from build123d import *
from OCP.BRepFilletAPI import BRepFilletAPI_MakeChamfer

# Parameters (mm, degrees)
SZKIC1_W                    = 47
SZKIC1_H                    = 33
SZKIC1_R                    = 7.6
DODANIE_WYCI_GNI_CIE1_DEPTH = 5
SZKIC2_W                    = 7
SZKIC2_H                    = 20.6
DODANIE_WYCI_GNI_CIE2_DEPTH = 10
SFAZOWANIE1_SIZE            = 5
SFAZOWANIE1_SIZE2           = 2.886751346
SZKIC3_R                    = 2
WYTNIJ_WYCI_GNI_CIE1_DEPTH  = 46.131917752
ZAOKR_GLENIE1_R             = 1
SZKIC4_W                    = 11.5
SZKIC4_H                    = 3
SZKIC4_W_2                  = 12
SZKIC4_H_2                  = 2.980259267
DODANIE_WYCI_GNI_CIE3_DEPTH = 27.5
DODANIE_WYCI_GNI_CIE4_START = 3
SZKIC5_W                    = 20.6
SZKIC5_H                    = 20.6
DODANIE_WYCI_GNI_CIE4_DEPTH = 3


with BuildPart() as part:
    # Szkic1 → Dodanie-wyciągnięcie1 (new body)
    # profile 1 of 3: a face of its own
    with BuildSketch(Plane.XY):
        Rectangle(SZKIC1_W, SZKIC1_H)
        Circle(SZKIC1_R, mode=Mode.SUBTRACT)
    # profile 2 of 3: a face of its own
    with BuildSketch(Plane.XY):
        with BuildLine():
            Line((4.175823272, -6.35), (-4.175823272, -6.35))
            ThreePointArc((-4.175823272, -6.35), (0, -7.6), (4.175823272, -6.35))
        make_face()
    # profile 3 of 3: a face of its own
    with BuildSketch(Plane.XY):
        with BuildLine():
            ThreePointArc((4.175823272, 6.35), (0, 7.6), (-4.175823272, 6.35))
            Line((-4.175823272, 6.35), (4.175823272, 6.35))
        make_face()
    extrude(amount=DODANIE_WYCI_GNI_CIE1_DEPTH)

    # Szkic2 → Dodanie-wyciągnięcie2 (add)
    with BuildSketch(Plane(origin=(0, 0, 0), x_dir=(-1, 0, 0), z_dir=(0, 0, -1))):
        with Locations((-13.8, 0)):
            Rectangle(SZKIC2_W, SZKIC2_H)
        with Locations((13.8, 0)):
            Rectangle(SZKIC2_W, SZKIC2_H)
    extrude(amount=DODANIE_WYCI_GNI_CIE2_DEPTH)

    # Sfazowanie1: one chamfer whose edges measure the first distance from different faces: ONE call of the kernel's chamfer builder (chamfer() names one face for all edges)
    sfazowanie1_edges_1 = [part.edges().sort_by_distance(p)[0] for p in [
        (13.8, 10.3, -10),
    ]]
    sfazowanie1_side_1 = [part.faces().sort_by_distance(p)[0] for p in [
        (13.8, 10.3, -5),
    ]]
    sfazowanie1_edges_2 = [part.edges().sort_by_distance(p)[0] for p in [
        (13.8, -10.3, -10),
    ]]
    sfazowanie1_side_2 = [part.faces().sort_by_distance(p)[0] for p in [
        (13.8, -10.3, -5),
    ]]
    sfazowanie1_edges_3 = [part.edges().sort_by_distance(p)[0] for p in [
        (-13.8, 10.3, -10),
    ]]
    sfazowanie1_side_3 = [part.faces().sort_by_distance(p)[0] for p in [
        (-13.8, 10.3, -5),
    ]]
    sfazowanie1_edges_4 = [part.edges().sort_by_distance(p)[0] for p in [
        (-13.8, -10.3, -10),
    ]]
    sfazowanie1_side_4 = [part.faces().sort_by_distance(p)[0] for p in [
        (-13.8, -10.3, -5),
    ]]
    sfazowanie1 = BRepFilletAPI_MakeChamfer(part.part.solid().wrapped)
    for e in sfazowanie1_edges_1:
        sfazowanie1.Add(SFAZOWANIE1_SIZE, SFAZOWANIE1_SIZE2, e.wrapped, sfazowanie1_side_1[0].wrapped)  # the first distance lies on this face
    for e in sfazowanie1_edges_2:
        sfazowanie1.Add(SFAZOWANIE1_SIZE, SFAZOWANIE1_SIZE2, e.wrapped, sfazowanie1_side_2[0].wrapped)  # the first distance lies on this face
    for e in sfazowanie1_edges_3:
        sfazowanie1.Add(SFAZOWANIE1_SIZE, SFAZOWANIE1_SIZE2, e.wrapped, sfazowanie1_side_3[0].wrapped)  # the first distance lies on this face
    for e in sfazowanie1_edges_4:
        sfazowanie1.Add(SFAZOWANIE1_SIZE, SFAZOWANIE1_SIZE2, e.wrapped, sfazowanie1_side_4[0].wrapped)  # the first distance lies on this face
    add(Compound.cast(sfazowanie1.Shape()), mode=Mode.REPLACE)

    # Szkic3 → Wytnij-wyciągnięcie1 (cut, through all)
    with BuildSketch(Plane(origin=(17.3, 0, 0), x_dir=(0, 0, -1), z_dir=(1, 0, 0))):
        with Locations((5, 4.3)):
            Circle(SZKIC3_R)
        with Locations((5, -4.3)):
            Circle(SZKIC3_R)
    extrude(amount=-WYTNIJ_WYCI_GNI_CIE1_DEPTH, mode=Mode.SUBTRACT)

    # Zaokrąglenie1
    zaokr_glenie1_edges = [part.edges().sort_by_distance(p)[0] for p in [
        (-23.5, -16.5, 2.5),
        (-23.5, 16.5, 2.5),
        (23.5, 16.5, 2.5),
        (23.5, -16.5, 2.5),
    ]]
    fillet(zaokr_glenie1_edges, radius=ZAOKR_GLENIE1_R)

    # Szkic4 → Dodanie-wyciągnięcie3 (add)
    with BuildSketch(Plane(origin=(0, 0, 0), x_dir=(-1, 0, 0), z_dir=(0, 0, -1))):
        with Locations((-1.5, 15)):
            Rectangle(SZKIC4_W, SZKIC4_H)
        with Locations((-1.25, -15.009870366)):
            Rectangle(SZKIC4_W_2, SZKIC4_H_2)
    extrude(amount=DODANIE_WYCI_GNI_CIE3_DEPTH)

    # Szkic5 → Dodanie-wyciągnięcie4 (add)
    with BuildSketch(Plane(origin=(0, 0, 0), x_dir=(-1, 0, 0), z_dir=(0, 0, -1)).offset(DODANIE_WYCI_GNI_CIE4_START)):
        Rectangle(SZKIC5_W, SZKIC5_H)
        with BuildLine():
            Line((4.175823272, -6.35), (-4.175823272, -6.35))
            ThreePointArc((-4.175823272, -6.35), (-7.6, 0), (-4.175823272, 6.35))
            Line((-4.175823272, 6.35), (4.175823272, 6.35))
            ThreePointArc((4.175823272, 6.35), (7.6, 0), (4.175823272, -6.35))
        make_face(mode=Mode.SUBTRACT)
    extrude(amount=-DODANIE_WYCI_GNI_CIE4_DEPTH)


solid = part.part
Geometry check sheet. Reference: the model listing, model coordinates, mm. A direction names the side the tool comes from. Round coordinates to 2 decimals unless told otherwise and drop trailing zeros. Order: outer loops, then holes, each group sorted by start corner. A loop starts at its lowest first (then second) coordinate and runs counter-clockwise, first axis right, second up. Notation, with made-up numbers: M 12.25,84.25 L 20.25,84.25 A9 ccw 20.25,100.25 Z; hole C 84,54.25 d9. An arc over 180 degrees is marked long. Answer in a Markdown table with one row per item. Add a question column.
Item 1: Sectioned sample at A-A, the plane z = -24.5. Enter the section's corners in (x, y), plus the area to 3 significant figures.
Item 2: Material ranges on L1, parallel to Y at x = 1, z = -11.5; L2, parallel to Z at x = 18.5, y = -12; L3, parallel to Z at x = 12, y = -7, recorded low to high. Write a range as [from, to].
Item 3: Sectioned sample at D-D, the plane z = 2.5. Enter the section's corners in (x, y), plus the area to 3 significant figures.
Item 4: Depth check by flat-ended pin: pin 1 Ø1 at (x, y) = (0.5, 9.5) entering from -Z; pin 2 Ø7.5 at (y, z) = (3, -7.5) entering from +X; pin 3 Ø2 at (x, y) = (15, 0.5) entering from -Z; pin 4 Ø2 at (y, z) = (5, -5) entering from -X. Enter the tip coordinate at first touch or a pass-through.
Item 5: Draft check along Y on faces 1 (the face through (-23.215, -16.199, 2.535)), 2 (the face through (0, -10.3, -2)), 3 (the face through (-23.5, 0, 2)). Enter one of: released by +Y, released by -Y, zero draft, split by the parting line, or undercut.
Item 6: Sectioned sample at B-B, the plane z = -1.5. Enter the section's corners in (x, y), plus the area to 3 significant figures.
Item 7: Sectioned sample at C-C, the plane x = 1.5. Enter the section's corners in (y, z).
Item 8: Set-up check for faces 4 (the face through (23.199, 16.215, 2.535)), 5 (the face through (0, 10.3, -2)), 6 (the face through (-4.25, 15, -14)): record each of +Z, -Z, +X, -X, +Y, -Y from which the full face is reachable in a straight line by a thin tool's end or side.
Filled in:
| question | item | result |
|---|---|---|
| 1 | outline | M -4.75,-16.5 L 7.25,-16.5 L 7.25,-13.52 L -4.75,-13.52 Z; M -4.25,13.5 L 7.25,13.5 L 7.25,16.5 L -4.25,16.5 Z |
| 1 | area | 70.3 mm² |
| 2 | L1 | y = [-16.5, -13.52], [13.5, 16.5] |
| 2 | L2 | z = [0, 5] |
| 2 | L3 | z = [-10, 5] |
| 3 | outline | M -23.5,-15.5 A1 ccw -22.5,-16.5 L 22.5,-16.5 A1 ccw 23.5,-15.5 L 23.5,15.5 A1 ccw 22.5,16.5 L -22.5,16.5 A1 ccw -23.5,15.5 Z; hole M -4.18,-6.35 L 4.18,-6.35 A7.6 ccw 4.18,6.35 L -4.18,6.35 A7.6 ccw Z |
| 3 | area | 1,380 mm² |
| 4 | pin 1 | stops at z = -3 |
| 4 | pin 2 | stops at x = 17.3 |
| 4 | pin 3 | stops at z = -10 |
| 4 | pin 4 | passes through |
| 5 | face 1 | released by -Y |
| 5 | face 2 | undercut |
| 5 | face 3 | zero draft |
| 6 | outline | M -17.3,-10.3 L 17.3,-10.3 L 17.3,10.3 L -17.3,10.3 Z; M -4.75,-16.5 L 7.25,-16.5 L 7.25,-13.52 L -4.75,-13.52 Z; M -4.25,13.5 L 7.25,13.5 L 7.25,16.5 L -4.25,16.5 Z; hole M -4.18,-6.35 L 4.18,-6.35 A7.6 ccw 4.18,6.35 L -4.18,6.35 A7.6 ccw Z |
| 6 | area | 616 mm² |
| 7 | outline | M -16.5,-27.5 L -13.52,-27.5 L -13.52,0 L -10.3,0 L -10.3,-3 L -6.35,-3 L -6.35,5 L -16.5,5 Z; M 6.35,-3 L 10.3,-3 L 10.3,0 L 13.5,0 L 13.5,-27.5 L 16.5,-27.5 L 16.5,5 L 6.35,5 Z |
| 8 | face 4 | +Z, -Z, +X, +Y |
| 8 | face 5 | -Z, +X, -X |
| 8 | face 6 | -Z, -X, +Y |
